Design review of the part shown in the three views and the two pictorial views. Dimensions are in mm from the part's minimum x, y and z. Round coordinates to 2 decimals unless told otherwise and drop trailing zeros. Loops run counter-clockwise (first coordinate to the right, second up) from the corner with the lowest first, then second, coordinate; pieces in that order, holes last. Notation, with made-up numbers: (29.5, 50.25) -> (62.5, 50.25) arc R19 cw to (62.5, 62.25) -> close; hole circle Ø6 at (-25.75, 53). An arc over 180 degrees is marked (long way). Use CSV: the item, a comma, the result in double quotes. Start each with the question number.
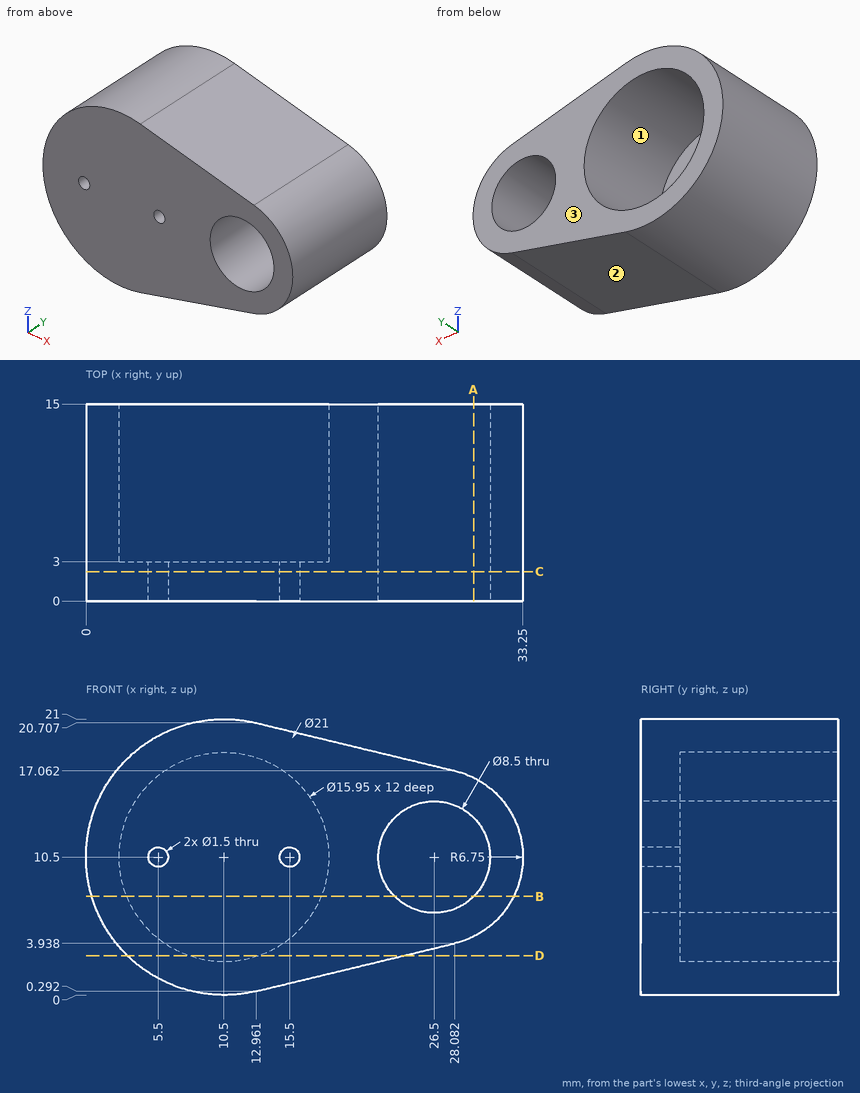
1. Take a section at A-A, the plane x = 29.5. Give the boundary of the cut face in (y, z).
2. The part is to be moulded in two halves that separate along X. For the marked faces 1, 2 and 3, say which applies: pulls with the +X half, pulls with the -X half, needs draft (parallel to the pull), parting line crosses it, or undercut.
3. Clearance check with flat-ended pins moving along their axes: P1, Ø3, axis at y = 10, z = 7, coming from the -X side; P2, Ø3, axis at y = 13, z = 8, coming from the -X side; P3, Ø3, axis at x = 29.5, y = 6, coming from the +Z side; P4, Ø0.9, axis at x = 5.5, z = 10.5, coming from the +Y side. State where each tip first meets the part, or that it passes through.
4. Take a section at B-B, the plane z = 7.5. Give the boundary of the cut face in (x, y), then the cut area to 3 significant figures.
5. Take a section at D-D, the plane z = 3. Give the boundary of the cut face in (x, y).
6. Take a section at C-C, the plane y = 2.25. Give the boundary of the cut face in (x, z).
7. For line 1 along X through (y, z) = (6, 12) (1 decimal); line 2 along Y through (x, z) = (10, 16.25); line 3 along X through (y, z) = (5.75, 15) (1 decimal), list the stretches that pass through material, from the lowest coordinate up. Write a range as from..to.
Results:
1,outline,"(0, 4.45) -> (15, 4.45) -> (15, 7.49) -> (0, 7.49) -> close; (0, 13.51) -> (15, 13.51) -> (15, 16.55) -> (0, 16.55) -> close"
2,face 1,"undercut"
2,face 2,"pulls with the +X half"
2,face 3,"needs draft"
3,P1,"x = 0.19"
3,P2,"x = 0.05"
3,P3,"z = 17.08"
3,P4,"through"
4,outline,"(0.44, 0) -> (23.49, 0) -> (23.49, 15) -> (17.89, 15) -> (17.89, 3) -> (3.11, 3) -> (3.11, 15) -> (0.44, 15) -> close; (29.51, 0) -> (32.55, 0) -> (32.55, 15) -> (29.51, 15) -> close"
4,area,"214 mm²"
5,outline,"(3.15, 0) -> (24.19, 0) -> (24.19, 15) -> (13.21, 15) -> (13.21, 3) -> (7.79, 3) -> (7.79, 15) -> (3.15, 15) -> close"
6,outline,"(12.96, 0.29) -> (28.08, 3.94) arc R6.75 ccw to (28.08, 17.06) -> (12.96, 20.71) arc R10.5 ccw (long way) to start; hole circle Ø1.5 at (5.5, 10.5); hole circle Ø1.5 at (15.5, 10.5); hole circle Ø8.5 at (26.5, 10.5)"
7,line 1,"0.1..2.7, 18.3..22.5, 30.5..33.1"
7,line 2,"0..3"
7,line 3,"1..3.9, 17.1..31.5"
